Design review of the part built by this model. Coordinates are the model's own, in mm. A direction names the side the tool comes from. Round coordinates to 2 decimals unless told otherwise and drop trailing zeros. Order: outer loops, then holes, each group sorted by start corner. A loop starts at its lowest first (then second) coordinate and runs counter-clockwise, first axis right, second up. Notation, with made-up numbers: M 43.25,14.25 L 88.25,14.25 A19 ccw 88.25,51.25 Z; hole C -25.5,82 d7. An arc over 180 degrees is marked long. Write item = value, one per line. Start each with the question number.
```python
from build123d import *

# Parameters (mm, degrees)
EXTRUDE_1_DEPTH     = 10
SKETCH_2_R          = 2.75
CUT_EXTRUDE_1_DEPTH = 60.160797831
SKETCH_3_R          = 2.75
CUT_EXTRUDE_2_DEPTH = 60.160797831
SKETCH_4_R          = 4
CUT_EXTRUDE_3_DEPTH = 26
SKETCH_5_R          = 4
CUT_EXTRUDE_4_DEPTH = 27


with BuildPart() as part:
    # 草图1 → 凸台-拉伸1 (new body)
    with BuildSketch(Plane.XY):
        Polygon((0, 0), (0, 50), (30, 0), align=None)
    extrude(amount=EXTRUDE_1_DEPTH)

    # 草图2 → 切除-拉伸1 (cut, through all)
    with BuildSketch(Plane.XZ):
        with Locations(Location((11, 5, 0), (0, 0, 270))):
            Circle(SKETCH_2_R)
    extrude(amount=-CUT_EXTRUDE_1_DEPTH, mode=Mode.SUBTRACT)

    # 草图3 → 切除-拉伸2 (cut, through all)
    with BuildSketch(Plane.ZY):
        with Locations((5, 40)):
            Circle(SKETCH_3_R)
    extrude(amount=-CUT_EXTRUDE_2_DEPTH, mode=Mode.SUBTRACT)

    # 草图4 → 切除-拉伸3 (cut)
    with BuildSketch(Plane(origin=(0, 50, 0), x_dir=(-1, 0, 0), z_dir=(0, -1, 0))):
        with Locations(Location((-11, -5, 0), (0, 0, 336.277210116))):
            Circle(SKETCH_4_R)
    extrude(amount=CUT_EXTRUDE_3_DEPTH, mode=Mode.SUBTRACT)

    # 草图5 → 切除-拉伸4 (cut)
    with BuildSketch(Plane.ZY.offset(-30)):
        with Locations(Location((5, 40, 0), (0, 0, 231.375167127))):
            Circle(SKETCH_5_R)
    extrude(amount=CUT_EXTRUDE_4_DEPTH, mode=Mode.SUBTRACT)


solid = part.part
```
(1) Consider section C-C, the plane x = 11. Write out the cut boundary in (y, z).
(2) Consider section D-D, the plane y = 8.5. Write out the cut boundary in (x, z).
(3) For line 1 along Z through (x, y) = (11, 27.5); line 2 along Y through (x, z) = (5, 7.5); line 3 along X through (y, z) = (16, 6.75), list the stretches that pass through material, from the lowest coordinate up. Write a range as [from, to].
(4) Draft analysis for pull direction Z (two halves, no side actions). For faces 1 (the face through (9, 14, 10)), 2 (the face through (3, 37, 4)), 3 (the face through (18, 20, 5)), state which applies: pulls with the +Z half, pulls with the -Z half, needs draft (parallel to the pull), parting line crosses it, or undercut.
(5) For faces 4 (the face through (13.32, 11.83, 3.52)), 5 (the face through (7, 29, 5)), 6 (the face through (4.93, 36.27, 3.56)), list the 3-axis set-ups (+Z, -Z, +X, -X, +Y, -Y) from which the entire face can be reached by the end or side of a thin tool; tool diameter is ignored.
(6) Consider section B-B, the plane z = 5. Write out the cut boundary in (x, y).
(7) Consider section A-A, the plane y = 40. Write out the cut boundary in (x, z).
(8) Insertion check: pin 1 (2 mm diameter, centred on y = 35, z = 8.5, fed in from +X); pin 2 (2.5 mm diameter, centred on x = 12.5, z = 6, fed in from +Y); pin 3 (4 mm diameter, centred on y = 40.5, z = 2, fed in from +X). Each pin has a flat end and moves straight along its axis. Give the tip position at first contact, or say it passes through.
Completed:
q1.outline = M 0,0 L 31.67,0 L 31.67,1 L 24,1 L 24,2.25 L 0,2.25 Z; M 0,7.75 L 24,7.75 L 24,9 L 31.67,9 L 31.67,10 L 0,10 Z
q2.outline = M 0,0 L 24.9,0 L 24.9,10 L 0,10 Z; hole C 11,5 d5.5
q3.line_1 = [0, 1], [9, 10]
q3.line_2 = [0, 36.88]
q3.line_3 = [0, 8.88], [13.12, 20.4]
q4.face_1 = pulls with the +Z half
q4.face_2 = undercut
q4.face_3 = needs draft
q5.face_4 = +Y, -Y
q5.face_5 = +Y
q5.face_6 = +X
q6.outline = M 0,0 L 8.25,0 L 8.25,24 L 7,24 L 7,36 L 3,36 L 3,37.25 L 0,37.25 Z; M 0,42.75 L 3,42.75 L 3,44 L 3.6,44 L 0,50 Z; M 13.75,0 L 30,0 L 15,25 L 15,24 L 13.75,24 Z
q7.outline = M 0,0 L 6,0 L 6,1 L 3,1 L 3,2.25 L 0,2.25 Z; M 0,7.75 L 3,7.75 L 3,9 L 6,9 L 6,10 L 0,10 Z
q8.pin_1 = 9.58
q8.pin_2 = 24
q8.pin_3 = 6.81
